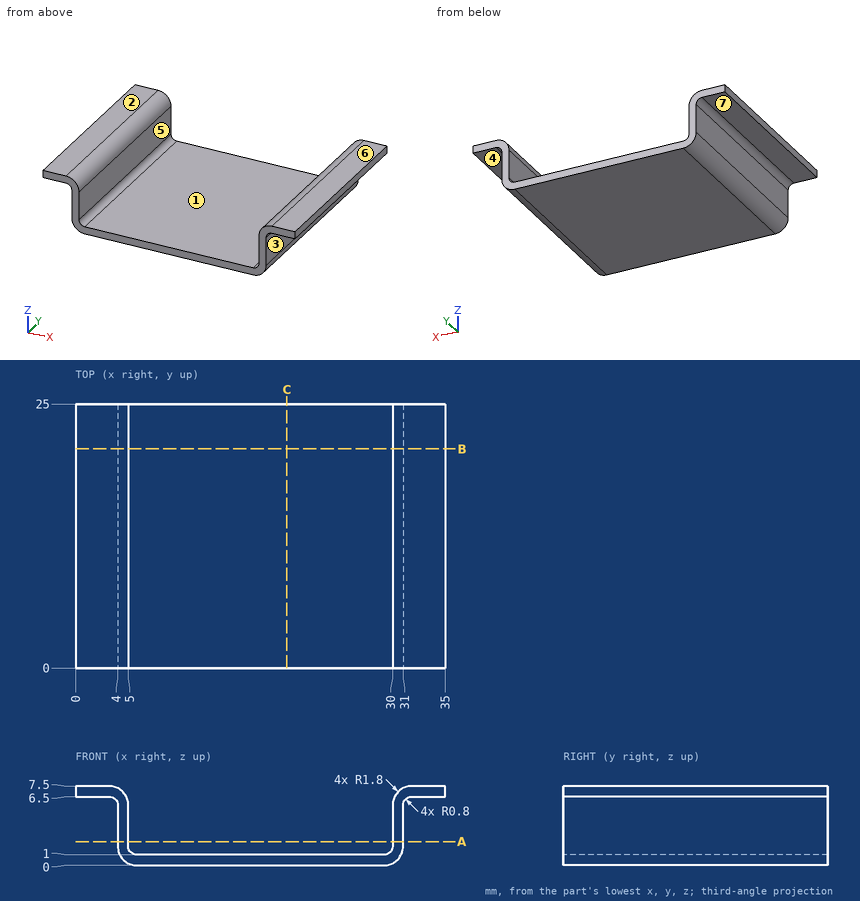
Verification items for this drawing (mm, ordinates from the low corner). A direction names the side the tool comes from. Coordinates: 2 decimals unless noted, no trailing zeros. Loops run counter-clockwise (first coordinate to the right, second up) from the corner with the lowest first, then second, coordinate; pieces in that order, holes last. Notation, with made-up numbers: (-28, -18) - (10, -18) arc R12 cw to (10, -8) - close; hole circle Ø5 at (79.25, 16.25). An arc over 180 degrees is marked (long way). Answer as a JSON object with one key per item and string values.
(1) Access from +Z, -Z, +X, -X, +Y, -Y to the whole of each face (thin tool, end or side, straight path). Record for the marked faces 4, 5, 6 and 7.
Response:
{"face 4": "-Z, +X, +Y, -Y", "face 5": "+Z, +Y, -Y", "face 6": "+Z, +X, -X, +Y, -Y", "face 7": "-Z, -X, +Y, -Y"}
(2) Cross-section at C-C, the plane x = 20. Record the boundary of the cut face in (y, z).
Response:
{"outline": "(0, 0) - (25, 0) - (25, 1) - (0, 1) - close"}
(3) Cross-section at B-B, the plane y = 20.75. Record the boundary of the cut face in (x, z).
Response:
{"outline": "(0, 6.5) - (3.2, 6.5) arc R0.8 cw to (4, 5.7) - (4, 1.8) arc R1.8 ccw to (5.8, 0) - (29.2, 0) arc R1.8 ccw to (31, 1.8) - (31, 5.7) arc R0.8 cw to (31.8, 6.5) - (35, 6.5) - (35, 7.5) - (31.8, 7.5) arc R1.8 ccw to (30, 5.7) - (30, 1.8) arc R0.8 cw to (29.2, 1) - (5.8, 1) arc R0.8 cw to (5, 1.8) - (5, 5.7) arc R1.8 ccw to (3.2, 7.5) - (0, 7.5) - close"}
(4) Scan lines: line 1 along X through (y, z) = (12.75, 4); line 2 along Z through (x, y) = (16, 5.75); line 3 along X through (y, z) = (5.25, 7) (3 decimals). Record each from-to range of solid material in increasing order.
Response:
{"line 1": "x = 4 to 5, 30 to 31", "line 2": "z = 0 to 1", "line 3": "x = 0 to 4.445, 30.555 to 35"}
(5) Mould release check, pull along X, two halves, no side actions. Record for the marked faces 1, 2 and 3: pulls with the +X half, pulls with the -X half, needs draft (parallel to the pull), parting line crosses it, or undercut.
Response:
{"face 1": "undercut", "face 2": "needs draft", "face 3": "pulls with the +X half"}
(6) Cross-section at A-A, the plane z = 2.25. Record the boundary of the cut face in (x, y), then the cut area to 3 significant figures.
Response:
{"outline": "(4, 0) - (5, 0) - (5, 25) - (4, 25) - close; (30, 0) - (31, 0) - (31, 25) - (30, 25) - close", "area": "50.0 mm²"}
(7) Go/stop test with flat-tipped pins: pin 1 Ø7 at (x, y) = (16.5, 6.5) entering from +Z; pin 2 Ø3.5 at (x, y) = (2, 8) entering from -Z; pin 3 Ø1.2 at (y, z) = (16, 4) entering from +X. Record where each tip stops, or that it passes through.
Response:
{"pin 1": "stops at z = 1", "pin 2": "stops at z = 6.28", "pin 3": "stops at x = 31"}
